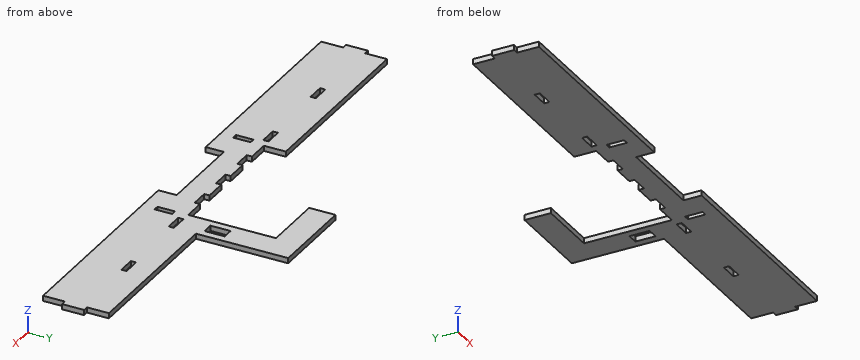
Solid Edge part; units mm, degrees
sketch "Sketch1" plane through (0, 0, 0) normal (0, 0, 1) x (1, 0, 0)
  line L0 (-110, 6.5) -> (-90, 6.5)
  line L1 (-90, 6.5) -> (-90, 12.5)
  line L2 (-110, 12.5) -> (-90, 12.5)
  line L3 (-110, 12.5) -> (-110, 6.5)
  line L4 (110, 142.5) -> (10, 142.5)
  line L5 (10, 142.5) -> (10, 112.5)
  line L6 (10, 112.5) -> (80, 112.5)
  line L7 (80, 112.5) -> (80, 75.5)
  line L8 (80, 75.5) -> (80, 12.5)
  line L9 (55, 12.5) -> (80, 12.5)
  line L10 (55, 6.5) -> (55, 12.5)
  line L11 (35, 6.5) -> (55, 6.5)
  line L12 (35, 12.5) -> (35, 6.5)
  line L13 (10, 12.5) -> (35, 12.5)
  line L14 (10, 6.5) -> (10, 12.5)
  line L15 (-10, 6.5) -> (10, 6.5)
  line L16 (-10, 12.5) -> (-10, 6.5)
  line L17 (-35, 12.5) -> (-10, 12.5)
  line L18 (-35, 6.5) -> (-35, 12.5)
  line L19 (-55, 6.5) -> (-35, 6.5)
  line L20 (-55, 12.5) -> (-55, 6.5)
  line L21 (-80, 12.5) -> (-55, 12.5)
  line L22 (-80, 37.5) -> (-80, 12.5)
  line L23 (-110, 37.5) -> (-80, 37.5)
  line L24 (-110, 37.5) -> (-294, 37.5)
  line L25 (-294, 12.5) -> (-294, 37.5)
  line L26 (-300, 12.5) -> (-294, 12.5)
  line L27 (-300, 12.5) -> (-300, -12.5)
  line L28 (-294, -12.5) -> (-300, -12.5)
  line L29 (-294, -37.5) -> (-294, -12.5)
  line L30 (-294, -37.5) -> (-50, -37.5)
  line L31 (-50, -16.7567) -> (-50, -37.5)
  line L32 (50, -16.7567) -> (-50, -16.7567)
  line L33 (50, -37.5) -> (50, -16.7567)
  line L34 (50, -37.5) -> (294, -37.5)
  line L35 (294, -12.5) -> (294, -37.5)
  line L36 (300, -12.5) -> (294, -12.5)
  line L37 (300, -12.5) -> (300, 12.5)
  line L38 (294, 12.5) -> (300, 12.5)
  line L39 (294, 37.5) -> (294, 12.5)
  line L40 (294, 37.5) -> (110, 37.5)
  line L41 (110, 37.5) -> (110, 75.5)
  line L42 (110, 112.5) -> (110, 75.5)
  line L43 (110, 112.5) -> (110, 142.5)
  line L44 (90, 6.5) -> (110, 6.5)
  line L45 (110, 6.5) -> (110, 12.5)
  line L46 (90, 12.5) -> (110, 12.5)
  line L47 (90, 12.5) -> (90, 6.5)
  line L48 (190, 6.5) -> (210, 6.5)
  line L49 (210, 6.5) -> (210, 12.5)
  line L50 (210, 12.5) -> (190, 12.5)
  line L51 (190, 12.5) -> (190, 6.5)
  line L52 (88.75, 42.5) -> (101.25, 42.5)
  line L53 (101.25, 42.5) -> (101.25, 65.5)
  line L54 (101.25, 65.5) -> (88.75, 65.5)
  line L55 (88.75, 65.5) -> (88.75, 42.5)
  line L56 (-80, -22.5) -> (-80, -2.5)
  line L57 (-80, -2.5) -> (-86, -2.5)
  line L58 (-86, -22.5) -> (-86, -2.5)
  line L59 (-86, -22.5) -> (-80, -22.5)
  line L60 (86, -22.5) -> (86, -2.5)
  line L61 (86, -2.5) -> (80, -2.5)
  line L62 (80, -22.5) -> (80, -2.5)
  line L63 (80, -22.5) -> (86, -22.5)
  line L64 (-210, 6.5) -> (-190, 6.5)
  line L65 (-190, 6.5) -> (-190, 12.5)
  line L66 (-190, 12.5) -> (-210, 12.5)
  line L67 (-210, 12.5) -> (-210, 6.5)
  dimension "D1" = 210
  dimension "D2" = 190
  dimension "D3" = 110
  dimension "D4" = 90
  dimension "D5" = 90
  dimension "D6" = 110
  dimension "D7" = 190
  dimension "D8" = 210
  dimension "D9" = 190
  dimension "D10" = 110
  dimension "D11" = 210
  dimension "D12" = 101.25
  dimension "D13" = 101.25
  dimension "D14" = 88.75
  dimension "D15" = 80
  dimension "D16" = 86
  dimension "D17" = 86
  dimension "D18" = 80
  dimension "D19" = 35
  dimension "D20" = 50
  dimension "D21" = 300
extrude "Protrusion1" add sketch "Sketch1" along normal blind 6
Read the model definition and answer for the solid it produces. Units are mm, in the model's axes. Give positions to 0.01 mm unless a question says otherwise; leave off trailing zeros. Write each loop counter-clockwise with the first axis right and the second up, starting at its lowest first coordinate (ties: lowest second). Pieces come first, ordered by that corner, then holes. Notation, with made-up numbers: M 88,-1 L 128,-1 A16 ccw 128,5 Z; hole C 5.5,87.25 d4. An arc over 180 degrees is marked long. One line per item, written item: value. Start each with the question number.
(1) Find section A-A (x = 73). Determine the outline of the cut face in (y, z), plus the area to 3 significant figures.
(2) Find section C-C (z = 4.15). Give the number of separate pieces and of enclosed holes in the cut face, plus the area to 3 significant figures.
(3) Find the intervals of material crossed by line 1 (X direction, y = -8, z = 0.85); line 2 (X direction, y = 32.5, z = 5.5); line 3 (X direction, y = 55, z = 5), in increasing order.
(4) Find section D-D (y = 100.5). Determine the outline of the cut face in (x, z).
(5) Flat-ended cylindrical pins translate along their axes: pin 1 Ø1.8 at (y, z) = (-27.5, 1.5) entering from +X; pin 2 Ø1.8 at (x, z) = (220, 4.5) entering from +Y; pin 3 Ø3 at (y, z) = (54, 4) entering from -X. Find the tip coordinate at first contact, or state that the pin passes through.
(6) Find section B-B (y = 18.5). Determine the outline of the cut face in (x, z), plus the area to 3 significant figures.
Results below:
1. outline: M -37.5,0 L 12.5,0 L 12.5,6 L -37.5,6 Z; M 112.5,0 L 142.5,0 L 142.5,6 L 112.5,6 Z
1. area: 480 mm^2
2. separate pieces: 1
2. enclosed holes: 7
2. area: 42,200 mm^2
3. line 1: x = -300 to -86, -80 to 80, 86 to 300
3. line 2: x = -294 to -80, 80 to 294
3. line 3: x = 80 to 88.75, 101.25 to 110
4. outline: M 80,0 L 110,0 L 110,6 L 80,6 Z
5. pin 1: stops at x = 294
5. pin 2: stops at y = 37.5
5. pin 3: stops at x = 80
6. outline: M -294,0 L -80,0 L -80,6 L -294,6 Z; M 80,0 L 294,0 L 294,6 L 80,6 Z
6. area: 2,570 mm^2
